Work out the finished part from the listing and answer in its coordinate system (mm). A direction names the side the tool comes from. Round coordinates to 2 decimals unless told otherwise and drop trailing zeros. Order: outer loops, then holes, each group sorted by start corner. A loop starts at its lowest first (then second) coordinate and runs counter-clockwise, first axis right, second up. Notation, with made-up numbers: (-19.75, 76.5) - (12.25, 76.5) arc R34 cw to (12.25, 109.5) - close; hole circle Ø5 at (20.25, -21.5). An arc over 180 degrees is marked (long way). Answer in a Markdown table with one row per item.
from build123d import *

# Parameters (mm, degrees)
SKETCH1_W           = 60
SKETCH1_H           = 40
BOSS_EXTRUDE3_DEPTH = 2.5
SKETCH3_R           = 10
SKETCH3_R_2         = 5
BOSS_EXTRUDE4_DEPTH = 20
FILLET7_R           = 5
SKETCH4_W           = 5
SKETCH4_H           = 40
BOSS_EXTRUDE6_DEPTH = 25
SKETCH5_W           = 40
SKETCH5_H           = 5
BOSS_EXTRUDE7_DEPTH = 20
FILLET8_R           = 5
FILLET9_R           = 10
FILLET10_R          = 15
SKETCH6_R           = 7.5
CUT_EXTRUDE1_DEPTH  = 20


with BuildPart() as part:
    # Sketch1 → Boss-Extrude3 (new, symmetric)
    with BuildSketch(Plane(origin=(0, 0, 0), x_dir=(1, 0, 0), z_dir=(0, 1, 0))):
        Rectangle(SKETCH1_W, SKETCH1_H)
    extrude(amount=BOSS_EXTRUDE3_DEPTH, both=True)

    # Sketch3 → Boss-Extrude4 (add, symmetric)
    with BuildSketch(Plane(origin=(0, 0, 0), x_dir=(1, 0, 0), z_dir=(0, 1, 0))):
        with Locations(Location((0, -20, 0), (0, 0, 270))):
            Circle(SKETCH3_R)
        with Locations(Location((0, -20, 0), (0, 0, 270))):
            Circle(SKETCH3_R_2, mode=Mode.SUBTRACT)
        with Locations(Location((0, 20, 0), (0, 0, 90))):
            Circle(SKETCH3_R)
        with Locations(Location((0, 20, 0), (0, 0, 90))):
            Circle(SKETCH3_R_2, mode=Mode.SUBTRACT)
    extrude(amount=BOSS_EXTRUDE4_DEPTH, both=True)

    # Fillet7
    fillet7_edges = [part.edges().sort_by_distance(p)[0] for p in [
        (0, 2.5, 10),
        (0, 2.5, -10),
    ]]
    fillet(fillet7_edges, radius=FILLET7_R)

    # Sketch4 → Boss-Extrude6 (add)
    with BuildSketch(Plane.XZ.offset(2.5)):
        with Locations((27.5, 0)):
            Rectangle(SKETCH4_W, SKETCH4_H)
        with Locations((-27.5, 0)):
            Rectangle(SKETCH4_W, SKETCH4_H)
    extrude(amount=BOSS_EXTRUDE6_DEPTH)

    # Sketch5 → Boss-Extrude7 (add)
    with BuildSketch(Plane(origin=(30, 0, 0), x_dir=(0, 0, -1), z_dir=(1, 0, 0))):
        with Locations((0, -25)):
            Rectangle(SKETCH5_W, SKETCH5_H)
    boss_extrude7 = extrude(amount=BOSS_EXTRUDE7_DEPTH)

    # Mirror1: Boss-Extrude7 across plane
    add(boss_extrude7.mirror(Plane(origin=(0, 0, 0), x_dir=(0, 0, 1), z_dir=(1, 0, 0))))

    # Fillet8
    fillet8_edges = [part.edges().sort_by_distance(p)[0] for p in [
        (30, -22.5, 0),
        (-30, -22.5, 0),
    ]]
    fillet(fillet8_edges, radius=FILLET8_R)

    # Fillet9
    fillet9_edges = [part.edges().sort_by_distance(p)[0] for p in [
        (25, -2.5, 0),
        (25, -27.5, 0),
        (-25, -2.5, 0),
        (-25, -27.5, 0),
    ]]
    fillet(fillet9_edges, radius=FILLET9_R)

    # Fillet10
    fillet10_edges = [part.edges().sort_by_distance(p)[0] for p in [
        (30, 2.5, 0),
        (-30, 2.5, 0),
    ]]
    fillet(fillet10_edges, radius=FILLET10_R)

    # Sketch6 → Cut-Extrude1 (cut)
    with BuildSketch(Plane(origin=(0, -22.5, 0), x_dir=(1, 0, 0), z_dir=(0, 1, 0))):
        with Locations((50, 0)):
            Circle(SKETCH6_R)
        with Locations((-50, 0)):
            Circle(SKETCH6_R)
    extrude(amount=-CUT_EXTRUDE1_DEPTH, mode=Mode.SUBTRACT)


solid = part.part
1) Find section A-A, the plane y = -15. Give the vertices of the cut face in (x, z), then the cut area to 3 significant figures.
Filled in:
| item | result |
|---|---|
| outline | (-30, -20) - (-25, -20) - (-25, 20) - (-30, 20) - close; circle Ø20 at (0, -20); circle Ø20 at (0, 20); (25, -20) - (30, -20) - (30, 20) - (25, 20) - close; hole circle Ø10 at (0, -20); hole circle Ø10 at (0, 20) |
| area | 871 mm^2 |
2) Each of these flat-tipped pins is pushed along its axis until it touches: pin 1 (8 mm diameter, centred on x = 17, z = 16.5, fed in from +Y); pin 2 (22 mm diameter, centred on x = 4.5, z = 16, fed in from -Y); pin 3 (12 mm diameter, centred on y = 12.5, z = -21, fed in from -X). Where does it stop, or does it pass through?
Filled in:
| item | result |
|---|---|
| pin 1 | stops at y = 2.78 |
| pin 2 | stops at y = -20 |
| pin 3 | stops at x = -10.08 |
3) The mould has two halves that part along X. Classify faces 5 (the face through (-30, -15, 0)), 6 (the face through (-42, -22.5, 0)), 7 (the face through (42.5, -24.96, -0.16)), 8 (the face through (1.5, 0.28, 24.77)): released by +X, released by -X, zero draft, split by the parting line, or undercut.
Filled in:
| item | result |
|---|---|
| face 5 | released by -X |
| face 6 | zero draft |
| face 7 | released by +X |
| face 8 | undercut |
4) Find section C-C, the plane z = 0. Give the vertices of the cut face in (x, y), then the cut area to 3 significant figures.
Filled in:
| item | result |
|---|---|
| outline | (-42.5, -27.5) - (-35, -27.5) arc R10 ccw to (-25, -17.5) - (-25, -12.5) arc R10 cw to (-15, -2.5) - (15, -2.5) arc R10 cw to (25, -12.5) - (25, -17.5) arc R10 ccw to (35, -27.5) - (42.5, -27.5) - (42.5, -22.5) - (35, -22.5) arc R5 cw to (30, -17.5) - (30, -12.5) arc R15 ccw to (15, 2.5) - (-15, 2.5) arc R15 ccw to (-30, -12.5) - (-30, -17.5) arc R5 cw to (-35, -22.5) - (-42.5, -22.5) - close |
| area | 589 mm^2 |
5) Find section B-B, the plane x = 0. Give the number of separate pieces and of enclosed holes in the cut face, then the cut area to 3 significant figures.
Filled in:
| item | result |
|---|---|
| separate pieces | 3 |
| enclosed holes | 0 |
| area | 961 mm^2 |
6) Find section D-D, the plane y = -7.5. Give the vertices of the cut face in (x, z).
Filled in:
| item | result |
|---|---|
| outline | (-29.14, -20) - (-23.66, -20) - (-23.66, 20) - (-29.14, 20) - close; circle Ø20 at (0, -20); circle Ø20 at (0, 20); (23.66, -20) - (29.14, -20) - (29.14, 20) - (23.66, 20) - close; hole circle Ø10 at (0, -20); hole circle Ø10 at (0, 20) |
7) Which of the six approach directions +Z, -Z, +X, -X, +Y, -Y give full straight-line access (tool end or side, diameter ignored) to faces 1 (the face through (28, -15, -20)), 2 (the face through (-1.5, -0.28, -24.77)), 3 (the face through (27.85, -24.49, 0.28)), 4 (the face through (28, -15, 20))?
Filled in:
| item | result |
|---|---|
| face 1 | -Z, +X, +Y, -Y |
| face 2 | none |
| face 3 | +Z, -Z, -Y |
| face 4 | +Z, +X, +Y, -Y |
8) Find the intervals of material crossed by probe 1 along X at (y, z) = (9, 20); probe 2 along X at (y, z) = (-6, -18); probe 3 along Y at (x, z) = (40, 6.5), in increasing order. Write a range as from..to.
Filled in:
| item | result |
|---|---|
| probe 1 | x = -10..-5, 5..10 |
| probe 2 | x = -28.52..-22.6, -9.8..-4.58, 4.58..9.8, 22.6..28.52 |
| probe 3 | y = -27.5..-22.5 |
